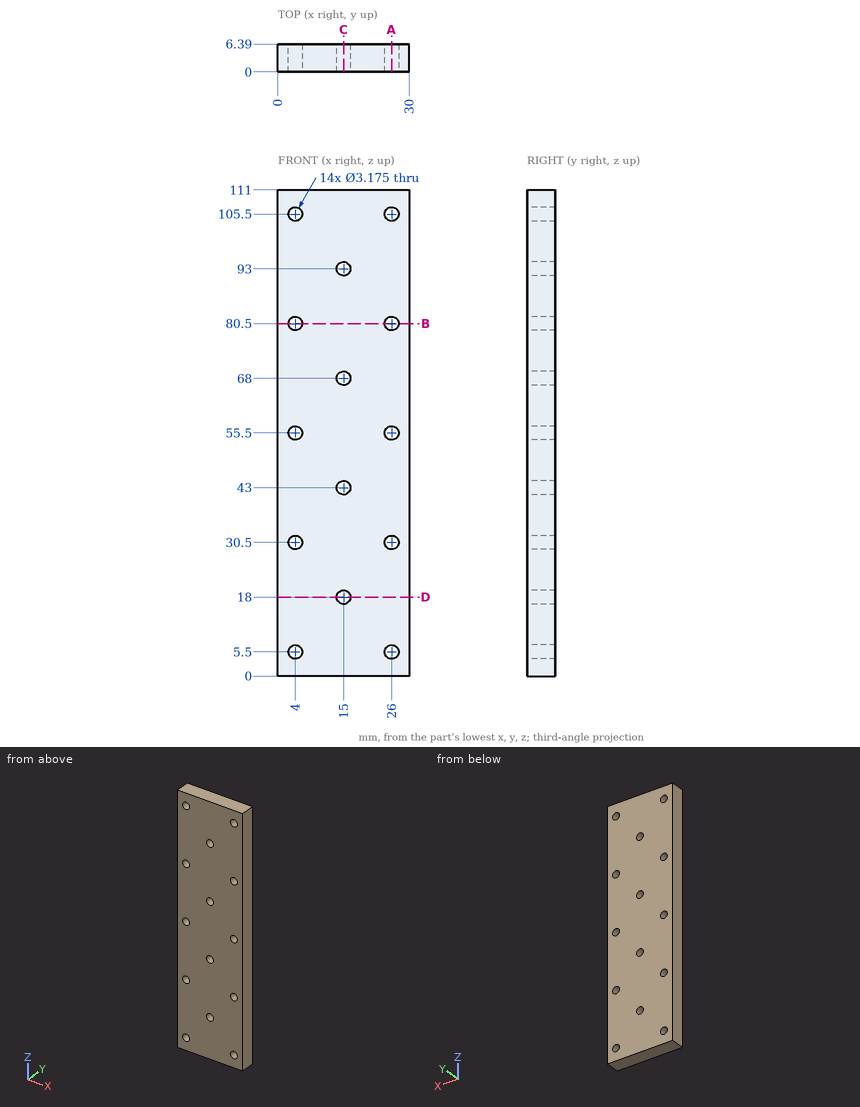
Geometry: see drawing. Coordinates: mm, zero at the bounding-box minimum. Give positions to 0.01 mm unless a question says otherwise; leave off trailing zeros. Order: outer loops, then holes, each group sorted by start corner. A loop starts at its lowest first (then second) coordinate and runs counter-clockwise, first axis right, second up. Notation, with made-up numbers: (-34, 61.25) -> (17, 61.25) arc R14 ccw to (17, 68.25) -> close; hole circle Ø7 at (55.5, 47). An arc over 180 degrees is marked (long way). Write each question's results on one line, items separated by ' | '. Start each with the question number.
1) Section D-D (z = 18). Return loops of the section in (x, y).
2) First-contact query: pin 1 (2.5 mm diameter, centred on x = 26, z = 5.5, fed in from -Y). Flat tip, straight axial feed; report the tip coordinate or a pass-through.
3) Section C-C (x = 15). Return loops of the section in (y, z).
4) Line query: line 1 (Z direction, x = 15, y = 3.75); line 2 (Z direction, x = 25.75, y = 6.25); line 3 (X direction, y = 3, z = 80.5). Output: solid intervals per line, ascending. Write a range as from..to.
5) Section A-A (x = 26). Return loops of the section in (y, z).
6) Section B-B (z = 80.5). Return loops of the section in (x, y), then the cut area to 3 significant figures.
Calculated:
1) outline: (0, 0) -> (13.41, 0) -> (13.41, 6.39) -> (0, 6.39) -> close; (16.59, 0) -> (30, 0) -> (30, 6.39) -> (16.59, 6.39) -> close
2) pin 1: through
3) outline: (0, 0) -> (6.39, 0) -> (6.39, 16.41) -> (0, 16.41) -> close; (0, 19.59) -> (6.39, 19.59) -> (6.39, 41.41) -> (0, 41.41) -> close; (0, 44.59) -> (6.39, 44.59) -> (6.39, 66.41) -> (0, 66.41) -> close; (0, 69.59) -> (6.39, 69.59) -> (6.39, 91.41) -> (0, 91.41) -> close; (0, 94.59) -> (6.39, 94.59) -> (6.39, 111) -> (0, 111) -> close
4) line 1: 0..16.41, 19.59..41.41, 44.59..66.41, 69.59..91.41, 94.59..111 | line 2: 0..3.93, 7.07..28.93, 32.07..53.93, 57.07..78.93, 82.07..103.93, 107.07..111 | line 3: 0..2.41, 5.59..24.41, 27.59..30
5) outline: (0, 0) -> (6.39, 0) -> (6.39, 3.91) -> (0, 3.91) -> close; (0, 7.09) -> (6.39, 7.09) -> (6.39, 28.91) -> (0, 28.91) -> close; (0, 32.09) -> (6.39, 32.09) -> (6.39, 53.91) -> (0, 53.91) -> close; (0, 57.09) -> (6.39, 57.09) -> (6.39, 78.91) -> (0, 78.91) -> close; (0, 82.09) -> (6.39, 82.09) -> (6.39, 103.91) -> (0, 103.91) -> close; (0, 107.09) -> (6.39, 107.09) -> (6.39, 111) -> (0, 111) -> close
6) outline: (0, 0) -> (2.41, 0) -> (2.41, 6.39) -> (0, 6.39) -> close; (5.59, 0) -> (24.41, 0) -> (24.41, 6.39) -> (5.59, 6.39) -> close; (27.59, 0) -> (30, 0) -> (30, 6.39) -> (27.59, 6.39) -> close | area: 151 mm2
